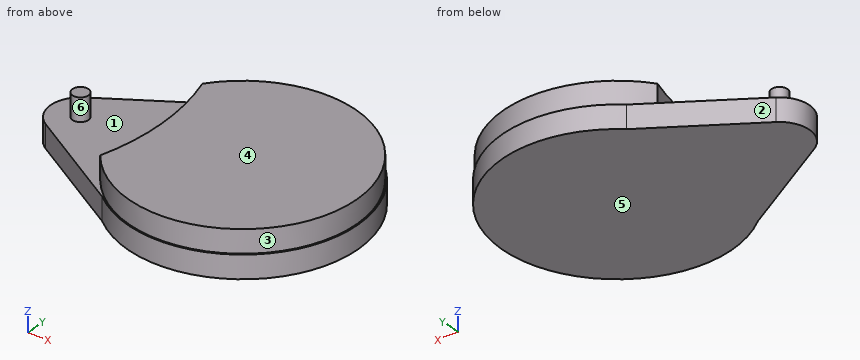
```python
from build123d import *

# Parameters (mm, degrees)
BOSS_EXTRUDE1_DEPTH = 5
SKETCH1_4_R         = 1.75
BOSS_EXTRUDE2_DEPTH = 5


with BuildPart() as part:
    # Sketch1 → Boss-Extrude1 (new body)
    with BuildSketch(Plane.XY):
        with BuildLine():
            ThreePointArc((29.416167617, 5.552080691), (26.296167617, 0), (29.416167617, -5.552080691))
            Line((29.416167617, -5.552080691), (51.653935363, -19.09000623))
            ThreePointArc((51.653935363, -19.09000623), (92.796167617, 0), (51.653935363, 19.09000623))
            Line((51.653935363, 19.09000623), (29.416167617, 5.552080691))
        make_face()
    extrude(amount=-BOSS_EXTRUDE1_DEPTH)

    # Sketch1_4 → Boss-Extrude2 (add)
    with BuildSketch(Plane.XY):
        with Locations((32.796167617, 0)):
            Circle(SKETCH1_4_R)
        with BuildLine():
            ThreePointArc((48.058176241, 14.849299526), (92.496167617, 0), (48.058176241, -14.849299526))
            ThreePointArc((48.058176241, -14.849299526), (50.3, 0), (48.058176241, 14.849299526))
        make_face()
    extrude(amount=BOSS_EXTRUDE2_DEPTH)


solid = part.part
```
Verification items for the finished model (mm, model axes). Face numbers are marked on the shaded views. A direction names the side the tool comes from. Coordinates: 2 decimals unless noted, no trailing zeros. Write each loop counter-clockwise with the first axis right and the second up, starting at its lowest first coordinate (ties: lowest second). Pieces come first, ordered by that corner, then holes. Notation, with made-up numbers: (16.25, 11.25) - (56.25, 11.25) arc R11 ccw to (56.25, 27.25) - close; hole circle Ø2 at (7.25, 65.5). An arc over 180 degrees is marked (long way). One line per question, with ' | ' between items. Start each with the question number.
1. Material ranges on line 1 along Z through (x, y) = (43.5, 6.5); line 2 along X through (y, z) = (1, 1.25); line 3 along X through (y, z) = (1.5, -1), recorded low to high.
2. Section check A-A (z = 3.5). Enter the section's corners in (x, y), plus the area to 3 significant figures.
3. Draft check along X on the marked faces 1, 2, 3 and 4. Enter one of: released by +X, released by -X, zero draft, split by the parting line, or undercut.
4. Access from +Z, -Z, +X, -X, +Y, -Y to the whole of each face (thin tool, end or side, straight path). Record for the marked faces 5 and 6.
5. Section check C-C (x = 80). Enter the section's corners in (y, z), plus the area to 3 significant figures.
6. Section check B-B (y = 0). Enter the section's corners in (x, z).
7. Section check D-D (z = -1.5). Enter the section's corners in (x, y), plus the area to 3 significant figures.
8. Gauge pin test, flat ends, axial feed: P1, Ø6, axis at y = 3, z = -1.5, coming from the -X side; P2, Ø6, axis at y = 17.5, z = 0, coming from the -X side; P3, Ø5, axis at x = 64.5, z = -1.5, coming from the -Y side; P4, Ø1, axis at x = 85.5, z = -3, coming from the +Y side. Record the tip position at first contact, or that the pin passes through.
Computed values:
1) line 1: -5 to 0 | line 2: 31.36 to 34.23, 50.29 to 92.48 | line 3: 26.47 to 92.75
2) outline: circle Ø3.5 at (32.8, 0); (48.06, -14.85) arc R24.7 ccw (long way) to (48.06, 14.85) arc R50.3 cw to start | area: 1,780 mm²
3) face 1: undercut | face 2: released by -X | face 3: split by the parting line | face 4: zero draft
4) face 5: -Z, +X, -X, +Y, -Y | face 6: +Z
5) outline: (-21.82, -5) - (21.82, -5) - (21.82, 0) - (21.47, 0) - (21.47, 5) - (-21.47, 5) - (-21.47, 0) - (-21.82, 0) - close | area: 433 mm²
6) outline: (26.3, -5) - (92.8, -5) - (92.8, 0) - (92.5, 0) - (92.5, 5) - (50.3, 5) - (50.3, 0) - (34.55, 0) - (34.55, 5) - (31.05, 5) - (31.05, 0) - (26.3, 0) - close
7) outline: (29.42, -5.55) - (51.65, -19.09) arc R25 ccw (long way) to (51.65, 19.09) - (29.42, 5.55) arc R6.5 ccw to start | area: 2,300 mm²
8) P1: x = 26.3 | P2: x = 44.11 | P3: y = -24.99 | P4: y = 18.14
